Part model, mm, in its own coordinate system. A direction names the side the tool comes from. Round coordinates to 2 decimals unless told otherwise and drop trailing zeros. Order: outer loops, then holes, each group sorted by start corner. A loop starts at its lowest first (then second) coordinate and runs counter-clockwise, first axis right, second up. Notation, with made-up numbers: (43, -23) -> (51, -23) arc R17 cw to (51, -8) -> close; hole circle Ø10 at (42, -36.75). An arc over 180 degrees is marked (long way). Use CSV: the item, a comma, the result in double quotes.
```python
from build123d import *

# Parameters (mm, degrees)
SKETCH17_W          = 90
SKETCH17_H          = 200
BOSS_EXTRUDE2_DEPTH = 200
CUT_EXTRUDE14_DEPTH = 200
FILLET1_R           = 10
SKETCH22_R          = 40
BOSS_EXTRUDE3_DEPTH = 5


with BuildPart() as part:
    # Loft5: read off the stored shape, not the designer's step
    # Loft5: loft between two sections, ruled curve by curve
    loft5_from = [
        Edge.make_bspline([(0, 9.572476569, 124.632931813), (0, -239.693387057, 143.777884951), (0, -258.838340195, -105.487978675), (0, -9.572476569, -124.632931813), (0, 239.693387057, -143.777884951), (0, 258.838340195, 105.487978675), (0, 9.572476569, 124.632931813)], [0, 0, 0, 0, 0.5, 0.5, 0.5, 1, 1, 1, 1], 3, [1, 0.333333333, 0.333333333, 1, 0.333333333, 0.333333333, 1]),
    ]
    loft5_to = [
        Edge.make_bspline([(500, 33.637216162, 94.172913775), (500, -154.708611388, 161.447346099), (500, -221.983043712, -26.898481451), (500, -33.637216162, -94.172913775), (500, 154.708611388, -161.447346099), (500, 221.983043712, 26.898481451), (500, 33.637216162, 94.172913775)], [0, 0, 0, 0, 0.5, 0.5, 0.5, 1, 1, 1, 1], 3, [1, 0.333333333, 0.333333333, 1, 0.333333333, 0.333333333, 1]),
    ]
    loft5 = Solid(Shell([*[Face.make_surface_from_curves(loft5_from[k], loft5_to[k]) for k in range(1)], Face(Wire(loft5_from)), Face(Wire(loft5_to))]))
    add(loft5)

    # Sketch17 → Boss-Extrude2 (add)
    with BuildSketch(Plane.ZY):
        with Locations((-2.678768884, 0)):
            Rectangle(SKETCH17_W, SKETCH17_H)
    extrude(amount=BOSS_EXTRUDE2_DEPTH)

    # Sketch21 → Cut-Extrude14 (cut)
    with BuildSketch(Plane(origin=(0, 0, -47.678768884), x_dir=(-1, 0, 0), z_dir=(0, 0, -1))):
        with BuildLine():
            Line((100, 100), (100, 139.740536385))
            Line((100, 139.740536385), (237.040054467, 139.740536385))
            Line((237.040054467, 139.740536385), (237.040054467, -127.442216689))
            Line((237.040054467, -127.442216689), (100, -127.442216689))
            Line((100, -127.442216689), (100, -100))
            ThreePointArc((100, -100), (200, 0), (100, 100))
        make_face()
    extrude(amount=-CUT_EXTRUDE14_DEPTH, mode=Mode.SUBTRACT)

    # Fillet1
    fillet1_edges = [part.edges().sort_by_distance(p)[0] for p in [
        (0, -9.572476569, -124.632931813),
    ]]
    fillet(fillet1_edges, radius=FILLET1_R)

    # Sketch22 → Boss-Extrude3 (add)
    with BuildSketch(Plane(origin=(500, 0, 0), x_dir=(0, 0, -1), z_dir=(1, 0, 0))):
        Circle(SKETCH22_R)
    extrude(amount=BOSS_EXTRUDE3_DEPTH)


solid = part.part
```
(1) Cut at A-A, the plane x = -64.5. Give the cut face in (y, z).
Reply:
outline,"(-100, -47.68) -> (100, -47.68) -> (100, 42.32) -> (-100, 42.32) -> close"
(2) Drop flat-ended pins along their axis: P1, Ø5, axis at x = 331.5, y = -17, coming from the +Z side; P2, Ø2, axis at x = 407, z = 39, coming from the -Y side; P3, Ø5, axis at x = 346.5, y = -94.5, coming from the +Z side. Give the stop position or say it passes through.
Reply:
P1,"z = 106.55"
P2,"y = -96.82"
P3,"z = 54.25"
(3) Which spindle directions (+Z, -Z, +X, -X, +Y, -Y) get a long thin tool onto all of the face, cutting with end or side? Do faces 1 (the face through (502.46, -39.05, 8.67)), 2 (the face through (-49, -100, -3)), 3 (the face through (-49, 100, -3)), 4 (the face through (-99, -1, -47.679)), 5 (the face through (-99, -1, 42.321)). Say none if no direction does.
Reply:
face 1,"+X"
face 2,"+Z, -Z, -X, -Y"
face 3,"+Z, -Z, -X, +Y"
face 4,"-Z, -X, +Y, -Y"
face 5,"+Z, -X, +Y, -Y"
